Read the model definition and answer for the solid it produces. Units are mm, in the model's axes. A direction names the side the tool comes from. Give positions to 0.01 mm unless a question says otherwise; leave off trailing zeros. Loops run counter-clockwise (first coordinate to the right, second up) from the corner with the lowest first, then second, coordinate; pieces in that order, holes last. Notation, with made-up numbers: (30, 4.5) -> (60, 4.5) arc R14 cw to (60, 9.5) -> close; hole circle Ø10 at (34.25, 44.25). An arc over 180 degrees is marked (long way). Answer as CSV lines item,"result". Start each with the question number.
Autodesk Inventor part; units mm, degrees
ref_plane "YZ Plane" through (0, 0, 0) normal (1, 0, 0) x (0, 1, 0)
ref_plane "XZ Plane" through (0, 0, 0) normal (0, 1, 0) x (-1, 0, 0)
ref_plane "XY Plane" through (0, 0, 0) normal (0, 0, 1) x (1, 0, 0)
sketch "Sketch1" plane through (0, 0, 0) normal (0, 1, 0) x (-1, 0, 0)
  point P0 (0, 0)
sketch "Sketch2" plane through (0, 0, 0) normal (0, 1, 0) x (-1, 0, 0)
  line L0 (3.95, 5.95) -> (-3.95, 5.95)
  line L1 (-3.95, 5.95) -> (-3.95, -5.95)
  line L2 (-3.95, -5.95) -> (3.95, -5.95)
  line L3 (3.95, -5.95) -> (3.95, 5.95)
  line L4 (3.95, 5.95) -> (-3.95, -5.95) construction
  line L5 (-3.95, 5.95) -> (3.95, -5.95) construction
  point P0 (0, 0)
  dimension "d0" = 7.9
  dimension "d1" = 11.9
extrude "Extrusion1" add sketch "Sketch2" against normal blind 4.5
fillet "Fillet1" radius 1.75 4 edges at (3.95, -2.25, 5.95) (3.95, -2.25, -5.95) (-3.95, -2.25, 5.95) (-3.95, -2.25, -5.95)
sketch "Sketch3" plane through (0, -4.5, 0) normal (0, -1, 0) x (1, 0, 0)
  line L0 (6, 6) -> (-6, 6)
  line L1 (-6, 6) -> (-6, -6)
  line L2 (-6, -6) -> (6, -6)
  line L3 (6, -6) -> (6, 6)
  line L4 (6, 6) -> (-6, -6) construction
  line L5 (-6, 6) -> (6, -6) construction
  point P0 (0, 0)
  dimension "d5" = 12
  dimension "d6" = 12
extrude "Extrusion2" add sketch "Sketch3" along normal blind 5.4
sketch "Sketch4" plane through (0, -9.9, 0) normal (0, -1, 0) x (1, 0, 0)
  line L0 (3.825, 3.825) -> (-3.825, 3.825)
  line L1 (-3.825, 3.825) -> (-3.825, -3.825)
  line L2 (-3.825, -3.825) -> (3.825, -3.825)
  line L3 (3.825, -3.825) -> (3.825, 3.825)
  line L4 (3.825, 3.825) -> (-3.825, -3.825) construction
  line L5 (-3.825, 3.825) -> (3.825, -3.825) construction
  point P0 (0, 0)
  dimension "d9" = 7.65
  dimension "d10" = 7.65
extrude "Extrusion3" cut sketch "Sketch4" against normal blind 4.4
properties part number "blank button_3DPrint"
(1) Find section D-D on z = 4.75. Write down the section's boundary in (x, y), then the cut area to 3 significant figures.
(2) Find section A-A on x = 3.25. Write down the section's boundary in (y, z) (3 decimals), then the cut area to 3 significant figures.
(3) Find section C-C on z = -1.5. Write down the section's boundary in (x, y) (3 decimals), then the cut area to 3 significant figures.
(4) The mould has two halves that part along X. Classify faces 1 (the face through (6, -7, 0)), 2 (the face through (3.825, -8, 0)), 3 (the face through (-3.451, -2.282, -5.424)): pulls with the +X half, pulls with the -X half, needs draft (parallel to the pull), parting line crosses it, or undercut.
(5) A tool of negligible diameter and unlimited length cuts with its end or side. For faces 4 (the face through (-3.825, -8, 0)), 5 (the face through (-3.95, -2, 0)), 6 (the face through (0, -2, 5.95)), 7 (the face through (-3.424, -2.282, 5.451)), from which of +Z, -Z, +X, -X, +Y, -Y can it reach the whole face along a straight path? Write none if from no direction.
(6) Each of these flat-tipped pins is pushed along its axis until it touches: P1, Ø4, axis at x = 3, z = -1.5, coming from the +Y side; P2, Ø2, axis at y = -2, z = -2, coming from the +X side; P3, Ø2, axis at x = 0, y = -2.5, coming from the +Z side; P4, Ø1, axis at x = -3, y = -2, coming from the -Z side. Where does it stop, or does it pass through?
(7) Find the intervals of material crossed by line 1 along X through (y, z) = (-6.5, 1) (3 decimals); line 2 along Y through (x, z) = (-4.5, 0.75), in increasing order. Write a range as from..to.
(8) Find section B-B on y = -3.5. Write down the section's boundary in (x, z).
Answer block:
1,outline,"(-6, -9.9) -> (6, -9.9) -> (6, -4.5) -> (3.86, -4.5) -> (3.86, 0) -> (-3.86, 0) -> (-3.86, -4.5) -> (-6, -4.5) -> close"
1,area,"99.6 mm2"
2,outline,"(-9.9, -6) -> (-4.5, -6) -> (-4.5, -5.6) -> (0, -5.6) -> (0, 5.6) -> (-4.5, 5.6) -> (-4.5, 6) -> (-9.9, 6) -> (-9.9, 3.825) -> (-5.5, 3.825) -> (-5.5, -3.825) -> (-9.9, -3.825) -> close"
2,area,"81.5 mm2"
3,outline,"(-6, -9.9) -> (-3.825, -9.9) -> (-3.825, -5.5) -> (3.825, -5.5) -> (3.825, -9.9) -> (6, -9.9) -> (6, -4.5) -> (3.95, -4.5) -> (3.95, 0) -> (-3.95, 0) -> (-3.95, -4.5) -> (-6, -4.5) -> close"
3,area,"66.7 mm2"
4,face 1,"pulls with the +X half"
4,face 2,"undercut"
4,face 3,"pulls with the -X half"
5,face 4,"-Y"
5,face 5,"+Z, -Z, -X, +Y"
5,face 6,"+Z, +X, -X, +Y"
5,face 7,"+Z, -X, +Y"
6,P1,"stops at y = 0"
6,P2,"stops at x = 3.95"
6,P3,"stops at z = 5.95"
6,P4,"stops at z = -5.92"
7,line 1,"x = -6..-3.825, 3.825..6"
7,line 2,"y = -9.9..-4.5"
8,outline,"(-3.95, -4.2) arc R1.75 ccw to (-2.2, -5.95) -> (2.2, -5.95) arc R1.75 ccw to (3.95, -4.2) -> (3.95, 4.2) arc R1.75 ccw to (2.2, 5.95) -> (-2.2, 5.95) arc R1.75 ccw to (-3.95, 4.2) -> close"
